Job drawing, mm, ordinate dimensions from the low corner. One solid piece. Coordinates: 2 decimals unless noted, no trailing zeros. Order: outer loops, then holes, each group sorted by start corner. A loop starts at its lowest first (then second) coordinate and runs counter-clockwise, first axis right, second up. Notation, with made-up numbers: M 1,3.25 L 32,3.25 A25 ccw 32,21.25 Z; hole C 78.5,77.5 d9. An arc over 180 degrees is marked long. Write item = value, one per line. Start each with the question number.
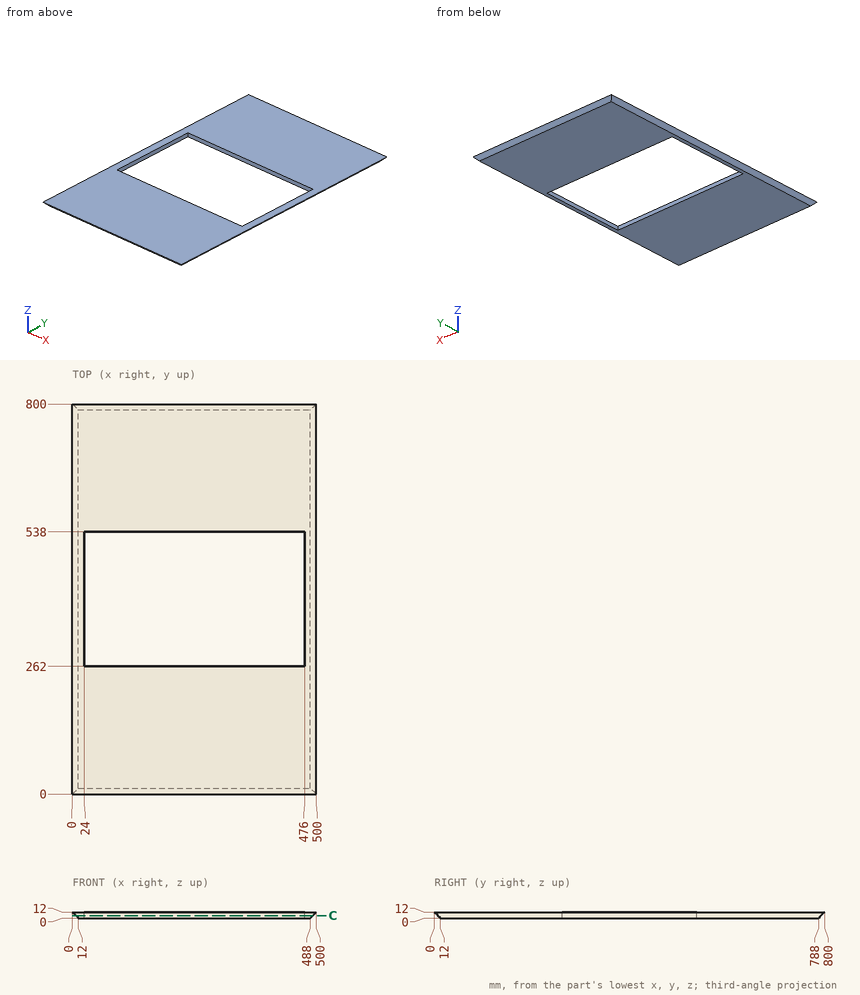
Item 1: Cut at C-C, the plane z = 4.75. Write the cut outline in (x, y).
Item 2: Flat gauge pins, fed straight in: pin 1 (3.5 mm diameter, centred on x = 315.5, z = 6.5, fed in from +Y); pin 2 (4 mm diameter, centred on x = 170, z = 5, fed in from -Y); pin 3 (1 mm diameter, centred on y = 269.5, z = 3, fed in from +X). Where does each tip first touch, or does it go through?
Item 3: Wall check: line 1 along Y through (x, z) = (366, 11.25); line 2 along X through (y, z) = (374, 6.25); line 3 along X through (y, z) = (415, 6.75). Give the ranges that are in metal, low to high. Write a range as [from, to].
Filled sheet:
q1.outline = M 7.25,7.25 L 492.75,7.25 L 492.75,792.75 L 7.25,792.75 Z; hole M 24,262 L 476,262 L 476,538 L 24,538 Z
q2.pin_1 = 796.25
q2.pin_2 = 5
q2.pin_3 = 491.5
q3.line_1 = [0.75, 262], [538, 799.25]
q3.line_2 = [5.75, 24], [476, 494.25]
q3.line_3 = [5.25, 24], [476, 494.75]
